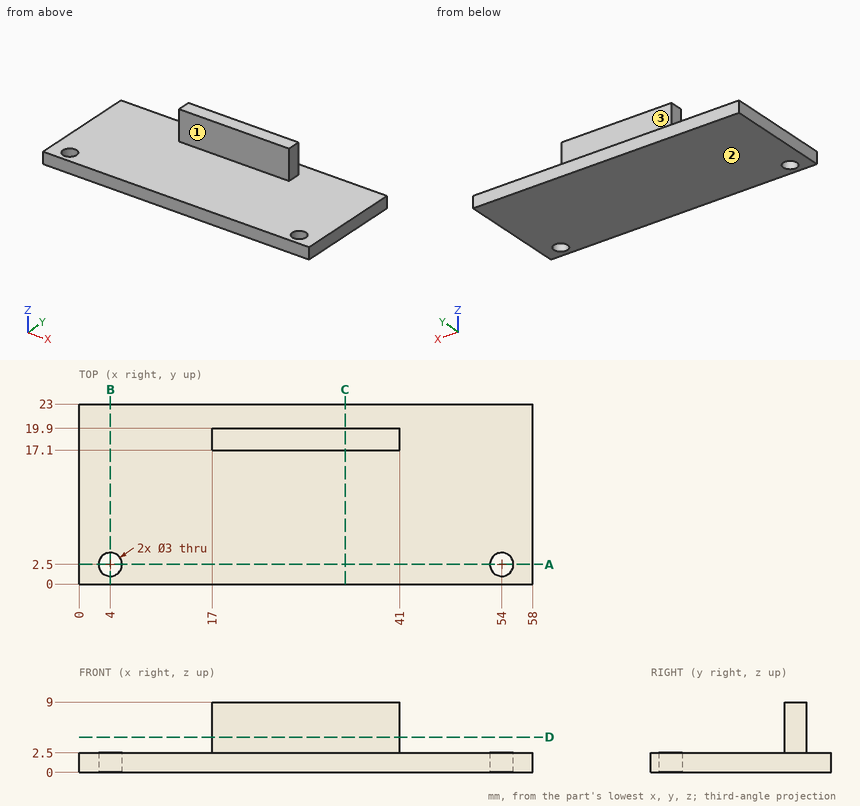
The figure shows three views and two pictorial views of one solid part (mm, origin at its lowest corner). Answer the questions. A direction names the side the tool comes from. Give positions to 0.01 mm unless a question says otherwise; leave off trailing zeros. Write each loop counter-clockwise with the first axis right and the second up, starting at its lowest first coordinate (ties: lowest second). Pieces come first, ordered by that corner, then holes. Notation, with made-up numbers: (66, 63) - (86, 63) arc R22 cw to (86, 98) - close; hole circle Ø2 at (24.25, 0). An arc over 180 degrees is marked (long way). Use CSV: the item, a comma, the result in double quotes. Start each with the question number.
Item 1: The part is cut by section D-D, the plane z = 4.5. Give the vertices of the cut face in (x, y).
Item 2: The part is cut by section B-B, the plane x = 4. Give the vertices of the cut face in (y, z).
Item 3: The part is cut by section A-A, the plane y = 2.5. Give the vertices of the cut face in (x, z).
Item 4: Flat-ended cylindrical pins translate along their axes: P1, Ø1, axis at y = 15, z = 7.5, coming from the +X side; P2, Ø2, axis at y = 18.5, z = 5, coming from the +X side; P3, Ø1, axis at y = 17.5, z = 7.5, coming from the -X side; P4, Ø1, axis at x = 25, y = 7.5, coming from the +Z side. Find the tip coordinate at first contact, or state that the pin passes through.
Item 5: Consider line 1 (Y direction, x = 4, z = 1.6); line 2 (Z direction, x = 3.5, y = 5.75); line 3 (Y direction, x = 32, z = 7). Determine where each line is inside the solid, lowest interval first.
Item 6: The part is cut by section C-C, the plane x = 34. Give the vertices of the cut face in (y, z).
Item 7: For the marked faces 1, 2 and 3, determine the directions among +Z, -Z, +X, -X, +Y, -Y from which every point of the face is accessible in a straight line to the end or side of a thin tool.
Taken from the geometry:
1,outline,"(17, 17.1) - (41, 17.1) - (41, 19.9) - (17, 19.9) - close"
2,outline,"(0, 0) - (1, 0) - (1, 2.5) - (0, 2.5) - close; (4, 0) - (23, 0) - (23, 2.5) - (4, 2.5) - close"
3,outline,"(0, 0) - (2.5, 0) - (2.5, 2.5) - (0, 2.5) - close; (5.5, 0) - (52.5, 0) - (52.5, 2.5) - (5.5, 2.5) - close; (55.5, 0) - (58, 0) - (58, 2.5) - (55.5, 2.5) - close"
4,P1,"through"
4,P2,"x = 41"
4,P3,"x = 17"
4,P4,"z = 2.5"
5,line 1,"0 to 1, 4 to 23"
5,line 2,"0 to 2.5"
5,line 3,"17.1 to 19.9"
6,outline,"(0, 0) - (23, 0) - (23, 2.5) - (19.9, 2.5) - (19.9, 9) - (17.1, 9) - (17.1, 2.5) - (0, 2.5) - close"
7,face 1,"+Z, +X, -X, -Y"
7,face 2,"-Z, +X, -X, +Y, -Y"
7,face 3,"+Z, +X, -X, +Y"
